Read the model definition and answer for the solid it produces. Units are mm, in the model's axes. Face numbers are marked on the shaded views. A direction names the side the tool comes from. Give positions to 0.01 mm unless a question says otherwise; leave off trailing zeros. Write each loop counter-clockwise with the first axis right and the second up, starting at its lowest first coordinate (ties: lowest second). Pieces come first, ordered by that corner, then holes.
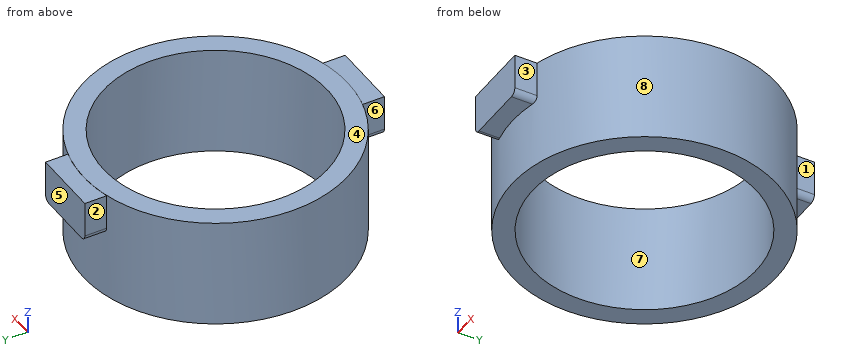
```python
from build123d import *

# Parameters (mm, degrees)
F0_R     = 11.15
F0_R_2   = 9.45
F1_DEPTH = 9.3
F3_W     = 5.7
F3_H     = 3.5
F4_DEPTH = 1.5
F5_R     = 0.5


with BuildPart() as f1:
    # F0 (on Top) → F1 (new body)
    with BuildSketch(Plane.XY):
        Circle(F0_R)
        Circle(F0_R_2, mode=Mode.SUBTRACT)
    extrude(amount=F1_DEPTH)

    # F3 (on offset) → F4 (join, symmetric)
    with BuildSketch(Plane.XZ.offset(11.15)):
        with Locations((0.0768768184, 7.5275215786)):
            Rectangle(F3_W, F3_H)
    extrude(amount=F4_DEPTH, both=True)

    # F5
    f5_edges = [f1.edges().sort_by_distance(p)[0] for p in [
        (-2.773123, -11.724821, 5.777522),
        (2.926877, -11.704496, 5.777522),
    ]]
    fillet(f5_edges, radius=F5_R)

    # F6: F1 across plane


with BuildPart() as f1_1:
    add(f1.part)
    add(f1.part.mirror(Plane.XZ))


solid = f1_1.part
```
Item 1: Find the intervals of material crossed by line 1 along Y through (x, z) = (0, 8.5); line 2 along Y through (x, z) = (0, 3.5); line 3 along X through (y, z) = (-6, 1), in increasing order.
Result set:
line 1: y = -12.65 to -9.45, 9.45 to 12.65
line 2: y = -11.15 to -9.45, 9.45 to 11.15
line 3: x = -9.4 to -7.3, 7.3 to 9.4
Item 2: Determine the mould class of the marked faces 6, 7 and 8 for opening direction Y: pulls with the +Y half, pulls with the -Y half, needs draft (parallel to the pull), parting line crosses it, or undercut.
Result set:
face 6: needs draft
face 7: undercut
face 8: parting line crosses it
Item 3: Each of these flat-tipped pins is pushed along its axis until it touches: pin 1 Ø0.9 at (y, z) = (11.5, 7.5) entering from +X; pin 2 Ø0.6 at (y, z) = (11.5, 8) entering from -X; pin 3 Ø0.9 at (x, y) = (1, 12) entering from -Z; pin 4 Ø11.5 at (x, y) = (0, 0) entering from +Z. Where does it stop, or does it pass through?
Result set:
pin 1: stops at x = 2.93
pin 2: stops at x = -2.77
pin 3: stops at z = 5.78
pin 4: passes through
Item 4: Section B-B (y = 0) is taken. Write down the section's boundary in (x, z).
Result set:
outline: (-11.15, 0) - (-9.45, 0) - (-9.45, 9.3) - (-11.15, 9.3) - close; (9.45, 0) - (11.15, 0) - (11.15, 9.3) - (9.45, 9.3) - close
Item 5: Section C-C (z = 8.25) is taken. Write down the section's boundary in (x, y), and give its area (3 significant figures).
Result set:
outline: (-2.77, -12.65) - (2.93, -12.65) - (2.93, -10.76) arc R11.15 ccw to (2.93, 10.76) - (2.93, 12.65) - (-2.77, 12.65) - (-2.77, 10.8) arc R11.15 ccw to (-2.77, -10.8) - close; hole circle Ø18.9 at (0, 0)
area: 129 mm2
Item 6: Which of the six approach directions +Z, -Z, +X, -X, +Y, -Y give full straight-line access (tool end or side, diameter ignored) to the marked faces 1, 2, 3, 4 and 5?
Result set:
face 1: +Z, -Z, +X, +Y
face 2: +Z, -Z, -X, +Y
face 3: +Z, -Z, +X, -Y
face 4: +Z, +X, -X, +Y, -Y
face 5: +Z, -Z, +X, -X, +Y
Item 7: Section D-D (y = -8.5) is taken. Write down the section's boundary in (x, z), and give its area (3 significant figures).
Result set:
outline: (-7.22, 0) - (-4.13, 0) - (-4.13, 9.3) - (-7.22, 9.3) - close; (4.13, 0) - (7.22, 0) - (7.22, 9.3) - (4.13, 9.3) - close
area: 57.4 mm2
